from build123d import *

# Parameters (mm, degrees)
F0_W         = 59.02
F0_H         = 32.4
F0_R         = 6.6906896399
F0_R_2       = 7.1640506352
F1_DEPTH     = 1.5
F2_W         = 5
F2_H         = 5
F3_DEPTH     = 6
F4_R         = 1
F5_R         = 1
F6_R         = 1.5
F7_T1_DEPTH  = 5.25
F7_S5_W      = 1.5
F7_S5_H      = 1.5
F7_T6_DEPTH  = 1.5
F7_S11_W     = 1.5
F7_S11_H     = 1.5
F7_T12_DEPTH = 1.5
F7_S17_W     = 1.5
F7_S17_H     = 1.5
F7_T18_DEPTH = 1.5
F7_S23_W     = 1.5
F7_S23_H     = 1.5
F7_T24_DEPTH = 1.5
F8_R         = 0.725
F9_DEPTH     = 35
F10_R        = 0.725
F11_DEPTH    = 35


# Not quite as in the source:
# - a fillet or chamfer that OpenCascade refuses, or shapes differently, is made with other operations: its cross-section is extruded or revolved along the edge and cut away or added


with BuildPart() as f1:
    # F0 (on Top) → F1 (new body, symmetric)
    with BuildSketch(Plane.XY):
        Rectangle(F0_W, F0_H)
        with Locations((-15.01, 0)):
            Circle(F0_R, mode=Mode.SUBTRACT)
        with Locations((15.01, 0)):
            Circle(F0_R_2, mode=Mode.SUBTRACT)
    extrude(amount=F1_DEPTH, both=True)

    # F2 (on face) → F3 (join)
    with BuildSketch(Plane.XY.offset(1.5)):
        with Locations((-23.76, -10.45)):
            Rectangle(F2_W, F2_H)
        with Locations((-23.76, 10.45)):
            Rectangle(F2_W, F2_H)
        with Locations((23.76, 10.45)):
            Rectangle(F2_W, F2_H)
        with Locations((23.76, -10.45)):
            Rectangle(F2_W, F2_H)
    extrude(amount=F3_DEPTH)

    # F4
    f4_edges = [f1.edges().sort_by_distance(p)[0] for p in [
        (26.26, -12.95, 4.5),
        (26.26, -7.95, 4.5),
        (26.26, 7.95, 4.5),
        (26.26, 12.95, 4.5),
        (21.26, -12.95, 4.5),
        (21.26, -7.95, 4.5),
        (-21.26, -12.95, 4.5),
        (-26.26, -12.95, 4.5),
        (-26.26, -7.95, 4.5),
        (-26.26, 7.95, 4.5),
        (-21.26, 7.95, 4.5),
        (21.26, 12.95, 4.5),
        (21.26, 7.95, 4.5),
        (-26.26, 12.95, 4.5),
        (-21.26, 12.95, 4.5),
        (-21.26, -7.95, 4.5),
    ]]
    fillet(f4_edges, radius=F4_R)

    # F5
    f5_edges = [f1.edges().sort_by_distance(p)[0] for p in [
        (-23.76, -7.95, 7.5),
        (-21.552893, -8.242893, 7.5),
        (-25.967107, -8.242893, 7.5),
        (-21.26, -10.45, 7.5),
        (-26.26, -10.45, 7.5),
        (-21.552893, -12.657107, 7.5),
        (-25.967107, -12.657107, 7.5),
        (-23.76, -12.95, 7.5),
        (-23.76, 12.95, 7.5),
        (-21.552893, 12.657107, 7.5),
        (-25.967107, 12.657107, 7.5),
        (-21.26, 10.45, 7.5),
        (-26.26, 10.45, 7.5),
        (-21.552893, 8.242893, 7.5),
        (-25.967107, 8.242893, 7.5),
        (-23.76, 7.95, 7.5),
        (23.76, 12.95, 7.5),
        (25.967107, 12.657107, 7.5),
        (21.552893, 12.657107, 7.5),
        (26.26, 10.45, 7.5),
        (21.26, 10.45, 7.5),
        (25.967107, 8.242893, 7.5),
        (21.552893, 8.242893, 7.5),
        (23.76, 7.95, 7.5),
        (23.76, -7.95, 7.5),
        (25.967107, -8.242893, 7.5),
        (21.552893, -8.242893, 7.5),
        (26.26, -10.45, 7.5),
        (21.26, -10.45, 7.5),
        (25.967107, -12.657107, 7.5),
        (21.552893, -12.657107, 7.5),
        (23.76, -12.95, 7.5),
        (7.845949, 0, 1.5),
        (-21.70069, 0, 1.5),
    ]]
    fillet(f5_edges, radius=F5_R)

    # F6
    f6_edges = [f1.edges().sort_by_distance(p)[0] for p in [
        (0, 16.2, -1.5),
        (-29.51, 0, -1.5),
        (0, -16.2, -1.5),
        (29.51, 0, -1.5),
    ]]
    fillet(f6_edges, radius=F6_R)

    # F7: fillet of radius 1.5 on 4 edges, made by hand

    # F7_s2 → F7_t1 (cut)
    with BuildSketch(Plane.XY):
        with BuildLine():
            ThreePointArc((29.51, 14.7), (29.0706601718, 15.7606601718), (28.01, 16.2))
            Line((28.01, 16.2), (29.51, 16.2))
            Line((29.51, 16.2), (29.51, 14.7))
        make_face()
        with BuildLine():
            ThreePointArc((-29.51, 14.7), (-29.0706601718, 15.7606601718), (-28.01, 16.2))
            Line((-28.01, 16.2), (-29.51, 16.2))
            Line((-29.51, 16.2), (-29.51, 14.7))
        make_face()
        with BuildLine():
            ThreePointArc((-28.01, -16.2), (-29.0706601718, -15.7606601718), (-29.51, -14.7))
            Line((-29.51, -14.7), (-29.51, -16.2))
            Line((-29.51, -16.2), (-28.01, -16.2))
        make_face()
        with BuildLine():
            ThreePointArc((28.01, -16.2), (29.0706601718, -15.7606601718), (29.51, -14.7))
            Line((29.51, -14.7), (29.51, -16.2))
            Line((29.51, -16.2), (28.01, -16.2))
        make_face()
    extrude(amount=F7_T1_DEPTH, mode=Mode.SUBTRACT)


with BuildPart() as f7_tool4:
    # F7_s5 → F7_t6 (new body)
    with BuildSketch(Plane.XZ.offset(14.7)):
        with Locations((28.76, -0.75)):
            Rectangle(F7_S5_W, F7_S5_H)
    extrude(amount=F7_T6_DEPTH)

    # F7_s7 → F7_t8 (revolve, cut)
    with BuildSketch(Plane(origin=(28.01, -14.7, 0), x_dir=(-0.7071067812, 0, 0.7071067812), z_dir=(0.7071067812, 0, 0.7071067812))):
        with BuildLine():
            ThreePointArc((0, -1.5), (1.5, 0), (0, 1.5))
            Line((0, 1.5), (0, -1.5))
        make_face()
    revolve(axis=Axis((28.01, -14.7, 0), (0, -1, 0)), mode=Mode.SUBTRACT)


with BuildPart() as f1_1:
    add(f1.part)

    # F7_t3: cut F7_tool4
    add(f7_tool4.part, mode=Mode.SUBTRACT)


with BuildPart() as f7_tool10:
    # F7_s11 → F7_t12 (new body)
    with BuildSketch(Plane.XZ.offset(14.7)):
        with Locations((-28.76, -0.75)):
            Rectangle(F7_S11_W, F7_S11_H)
    extrude(amount=F7_T12_DEPTH)

    # F7_s13 → F7_t14 (revolve, cut)
    with BuildSketch(Plane(origin=(-28.01, -14.7, 0), x_dir=(0.7071067812, 0, 0.7071067812), z_dir=(0.7071067812, 0, -0.7071067812))):
        with BuildLine():
            ThreePointArc((0, -1.5), (1.5, 0), (0, 1.5))
            Line((0, 1.5), (0, -1.5))
        make_face()
    revolve(axis=Axis((-28.01, -14.7, 0), (0, -1, 0)), mode=Mode.SUBTRACT)


with BuildPart() as f1_2:
    add(f1_1.part)

    # F7_t9: cut F7_tool10
    add(f7_tool10.part, mode=Mode.SUBTRACT)


with BuildPart() as f7_tool16:
    # F7_s17 → F7_t18 (new body)
    with BuildSketch(Plane.YZ.offset(-28.01)):
        with Locations((15.45, -0.75)):
            Rectangle(F7_S17_W, F7_S17_H)
    extrude(amount=-F7_T18_DEPTH)

    # F7_s19 → F7_t20 (revolve, cut)
    with BuildSketch(Plane(origin=(-28.01, 14.7, 0), x_dir=(0, -0.7071067812, 0.7071067812), z_dir=(0, -0.7071067812, -0.7071067812))):
        with BuildLine():
            ThreePointArc((0, -1.5), (1.5, 0), (0, 1.5))
            Line((0, 1.5), (0, -1.5))
        make_face()
    revolve(axis=Axis((-28.01, 14.7, 0), (-1, 0, 0)), mode=Mode.SUBTRACT)


with BuildPart() as f1_3:
    add(f1_2.part)

    # F7_t15: cut F7_tool16
    add(f7_tool16.part, mode=Mode.SUBTRACT)


with BuildPart() as f7_tool22:
    # F7_s23 → F7_t24 (new body)
    with BuildSketch(Plane.YZ.offset(28.01)):
        with Locations((15.45, -0.75)):
            Rectangle(F7_S23_W, F7_S23_H)
    extrude(amount=F7_T24_DEPTH)

    # F7_s25 → F7_t26 (revolve, cut)
    with BuildSketch(Plane(origin=(28.01, 14.7, 0), x_dir=(0, -0.7071067812, 0.7071067812), z_dir=(0, 0.7071067812, 0.7071067812))):
        with BuildLine():
            ThreePointArc((0, -1.5), (1.5, 0), (0, 1.5))
            Line((0, 1.5), (0, -1.5))
        make_face()
    revolve(axis=Axis((28.01, 14.7, 0), (1, 0, 0)), mode=Mode.SUBTRACT)


with BuildPart() as f1_4:
    add(f1_3.part)

    # F7_t21: cut F7_tool22
    add(f7_tool22.part, mode=Mode.SUBTRACT)

    # F8 (on face) → F9 (cut)
    with BuildSketch(Plane.XZ.offset(12.95)):
        with Locations((23.76, 4)):
            Circle(F8_R)
    extrude(amount=-F9_DEPTH, mode=Mode.SUBTRACT)

    # F10 (on face) → F11 (cut)
    with BuildSketch(Plane.XZ.offset(12.95)):
        with Locations((-23.76, 4)):
            Circle(F10_R)
    extrude(amount=-F11_DEPTH, mode=Mode.SUBTRACT)


solid = f1_4.part
Work out the finished part from the listing and answer in its coordinate system (mm). A direction names the side the tool comes from. Round coordinates to 2 decimals unless told otherwise and drop trailing zeros. Write each loop counter-clockwise with the first axis right and the second up, starting at its lowest first coordinate (ties: lowest second). Pieces come first, ordered by that corner, then holes.
1) A cutting plane is placed at D-D (x = -15.01). Give the vertices of the cut face in (y, z).
2) A tool of negligible diameter and unlimited length cuts with its end or side. For faces 5 (the flat face through (-24, -12.95, 5)), 6 (the flat face through (26.26, -10, 4)), 7 (the flat face through (-21.26, -10, 4)), 8 (the flat face through (24, -7.95, 5)), from which of +Z, -Z, +X, -X, +Y, -Y can it reach the whole face along a straight path? Write none if from no direction.
3) A cutting plane is placed at B-B (y = -10.5). Give the vertices of the cut face in (x, z) (3 decimals).
4) A cutting plane is placed at C-C (x = 23.76). Give the vertices of the cut face in (y, z) (3 decimals).
5) Straight lines are drawn through the part: line 1 (Z direction, x = -23.76, y = 11.55) (3 decimals); line 2 (X direction, y = 8.5, z = 4.5) (3 decimals); line 3 (Z direction, x = 27.5, y = 0.5). For each, find the intervals that lie inside material, in ascending order.
6) Given pin 1 Ø2.5 at (x, z) = (-24, 3) entering from -Y; pin 2 Ø12 at (x, y) = (16, 10) entering from +Z; pin 3 Ø5 at (x, y) = (2.5, -1) entering from +Z, each flat-ended and moving along its own axis, determine where each tip first touches the part or whether it passes through.
7) A cutting plane is placed at A-A (x = 15.01). Give the vertices of the cut face in (y, z), plus the area to 3 significant figures.
8) The mould has two halves that part along Z. Classify faces 1 (the cylindrical face through (29.08, 15.75, 0.74)), 2 (the flat face through (0, 0, -1.5)), 3 (the cylindrical face through (-23.1, 10.4, 3.7)), 4 (the flat face through (-24, 10, 7.5)): pulls with the +Z half, pulls with the -Z half, needs draft (parallel to the pull), parting line crosses it, or undercut.
Completed:
1. outline: (-16.2, 0) arc R1.5 ccw to (-14.7, -1.5) - (-6.69, -1.5) - (-6.69, 0.5) arc R1 ccw to (-7.69, 1.5) - (-16.2, 1.5) - close; (6.69, -1.5) - (14.7, -1.5) arc R1.5 ccw to (16.2, 0) - (16.2, 1.5) - (7.69, 1.5) arc R1 ccw to (6.69, 0.5) - close
2. face 5: +Z, +X, -X, -Y
2. face 6: +Z, +X, +Y, -Y
2. face 7: +Z, +Y, -Y
2. face 8: +Z, +X, -X
3. outline: (-29.51, 0) arc R1.5 ccw to (-28.01, -1.5) - (28.01, -1.5) arc R1.5 ccw to (29.51, 0) - (29.51, 1.5) - (26.26, 1.5) - (26.26, 6.5) arc R1 ccw to (25.26, 7.5) - (22.26, 7.5) arc R1 ccw to (21.26, 6.5) - (21.26, 1.5) - (-21.26, 1.5) - (-21.26, 6.5) arc R1 ccw to (-22.26, 7.5) - (-25.26, 7.5) arc R1 ccw to (-26.26, 6.5) - (-26.26, 1.5) - (-29.51, 1.5) - close; hole circle Ø1.45 at (-23.76, 4); hole circle Ø1.45 at (23.76, 4)
4. outline: (-16.2, 0) arc R1.5 ccw to (-14.7, -1.5) - (14.7, -1.5) arc R1.5 ccw to (16.2, 0) - (16.2, 1.5) - (12.95, 1.5) - (12.95, 3.275) - (7.95, 3.275) - (7.95, 1.5) - (-7.95, 1.5) - (-7.95, 3.275) - (-12.95, 3.275) - (-12.95, 1.5) - (-16.2, 1.5) - close; (-12.95, 4.725) - (-7.95, 4.725) - (-7.95, 6.5) arc R1 ccw to (-8.95, 7.5) - (-11.95, 7.5) arc R1 ccw to (-12.95, 6.5) - close; (7.95, 4.725) - (12.95, 4.725) - (12.95, 6.5) arc R1 ccw to (11.95, 7.5) - (8.95, 7.5) arc R1 ccw to (7.95, 6.5) - close
5. line 1: z = -1.5 to 3.275, 4.725 to 7.5
5. line 2: x = -26.153 to -24.285, -23.235 to -21.367, 21.367 to 23.235, 24.285 to 26.153
5. line 3: z = -1.5 to 1.5
6. pin 1: stops at y = -12.95
6. pin 2: stops at z = 7.47
6. pin 3: stops at z = 1.5
7. outline: (-16.2, 0) arc R1.5 ccw to (-14.7, -1.5) - (-7.16, -1.5) - (-7.16, 0.5) arc R1 ccw to (-8.16, 1.5) - (-16.2, 1.5) - close; (7.16, -1.5) - (14.7, -1.5) arc R1.5 ccw to (16.2, 0) - (16.2, 1.5) - (8.16, 1.5) arc R1 ccw to (7.16, 0.5) - close
7. area: 52.8 mm2
8. face 1: needs draft
8. face 2: pulls with the -Z half
8. face 3: undercut
8. face 4: pulls with the +Z half
